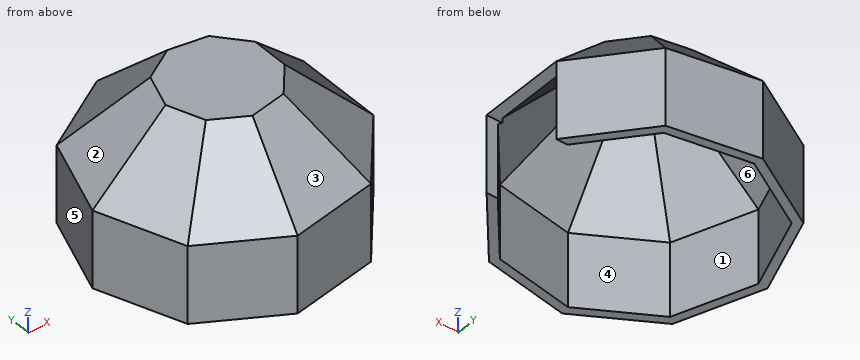
from build123d import *

# Parameters (mm, degrees)
F1_DEPTH = 85
F2_SIZE  = 40
F3_T     = -5
F4_W     = 50.557665
F4_H     = 45
F5_DEPTH = 70


with BuildPart() as f1:
    # F0 (on Top) → F1 (new body)
    with BuildSketch(Plane.XY):
        Polygon((-4.485587, -1.35111), (-4.485587, 49.206555), (-36.983427, 87.935973), (-86.773008, 96.715219), (-130.55723, 71.436387), (-147.84897, 23.927722), (-130.55723, -23.580943), (-86.773008, -48.859775), (-36.983427, -40.080529), align=None)
    extrude(amount=F1_DEPTH)

    # F2
    f2_edges = [f1.edges().sort_by_distance(p)[0] for p in [
        (-20.734507, -20.71582, 85),
        (-4.485587, 23.927722, 85),
        (-20.734507, 68.571264, 85),
        (-61.878218, 92.325596, 85),
        (-108.665119, 84.075803, 85),
        (-139.2031, 47.682054, 85),
        (-139.2031, 0.17339, 85),
        (-108.665119, -36.220359, 85),
        (-61.878218, -44.470152, 85),
    ]]
    chamfer(f2_edges, length=F2_SIZE)

    # F3
    f3_openings = [f1.faces().sort_by_distance(p)[0] for p in [
        (-73.938608, 23.927722, 0),
    ]]
    offset(amount=F3_T, openings=f3_openings)

    # F4 (on face) → F5 (cut)
    with BuildSketch(Plane.YZ.offset(-4.485587)):
        with Locations((23.927722, 22.5)):
            Rectangle(F4_W, F4_H)
    extrude(amount=-F5_DEPTH, mode=Mode.SUBTRACT)


solid = f1.part
Could you check a few things on this model? Use its own coordinates, in mm. Face numbers are marked on the shaded views. A direction names the side the tool comes from. Round coordinates to 2 decimals unless told otherwise and drop trailing zeros. Write each loop counter-clockwise with the first axis right and the second up, starting at its lowest first coordinate (ties: lowest second). Pieces come first, ordered by that corner, then holes. Notation, with made-up numbers: (4.5, 57.5) - (59.5, 57.5) arc R5 cw to (59.5, 61.5) - close; hole circle Ø11 at (88.5, -19.5). An arc over 180 degrees is marked (long way). Use a Markdown table: item, result.
Q1. I want a section at A-A (z = 64). List the corners of the cut face in (x, y) for me.
Output values:
| item | result |
|---|---|
| outline | (-127.63, 23.93) - (-115.07, -10.58) - (-83.26, -28.95) - (-47.09, -22.57) - (-23.49, 5.56) - (-23.49, 42.29) - (-47.09, 70.43) - (-83.26, 76.8) - (-115.07, 58.44) - close; hole (-120.1, 23.93) - (-109.3, -5.75) - (-81.96, -21.54) - (-50.86, -16.05) - (-30.56, 8.14) - (-30.56, 39.72) - (-50.86, 63.91) - (-81.96, 69.39) - (-109.3, 53.6) - close |
Q2. I want a section at C-C (z = 6.5). List the corners of the cut face in (x, y) for me, plus the area to 3 significant figures.
Output values:
| item | result |
|---|---|
| outline | (-147.85, 23.93) - (-130.56, -23.58) - (-86.77, -48.86) - (-36.98, -40.08) - (-4.49, -1.35) - (-11.01, -1.35) - (-39.64, -35.47) - (-85.85, -43.62) - (-126.48, -20.16) - (-142.53, 23.93) - (-126.48, 68.02) - (-85.85, 91.48) - (-39.64, 83.33) - (-11.01, 49.21) - (-4.49, 49.21) - (-36.98, 87.94) - (-86.77, 96.72) - (-130.56, 71.44) - close |
| area | 1,940 mm2 |
Q3. Thinking about a two-plate mould opening in Y: for the marked faces 1, 2, 3 and 4, which applies, released by +Y, released by -Y, zero draft, split by the parting line, or undercut?
Output values:
| item | result |
|---|---|
| face 1 | undercut |
| face 2 | released by +Y |
| face 3 | released by -Y |
| face 4 | undercut |
Q4. For pin 1 (6 mm diameter, centred on x = -48.5, z = 60, fed in from +Y); pin 2 (4 mm diameter, centred on x = -113, z = 17, fed in from -Y); pin 3 (8 mm diameter, centred on x = -104.5, y = 31, fed in from -Z), each with a flat end and sliding along its axis, tell me the tip position at first contact or that it passes through.
Output values:
| item | result |
|---|---|
| pin 1 | y = 77.83 |
| pin 2 | y = -34.87 |
| pin 3 | z = 72.24 |
Q5. Please list where these lines run through material, in increasing order: L1, parallel to Y at x = -91, z = 34; L2, parallel to X at y = -17, z = 5; L3, parallel to Y at x = -64.5, z = 61.
Output values:
| item | result |
|---|---|
| L1 | -46.42 to -40.65, 88.5 to 94.27 |
| L2 | -132.95 to -127.63, -24.14 to -17.62 |
| L3 | -28.69 to -21.51, 69.36 to 76.54 |
Q6. For the marked faces 5 and 6, which set-ups out of +Z, -Z, +X, -X, +Y, -Y let a thin tool reach every point of the face, with its end or its side?
Output values:
| item | result |
|---|---|
| face 5 | +Z, -Z, -X, +Y |
| face 6 | -Z |
Q7. I want a section at D-D (x = -67.5). List the corners of the cut face in (y, z) for me.
Output values:
| item | result |
|---|---|
| outline | (-45.46, 0) - (-40.38, 0) - (-40.38, 42.93) - (-2.74, 80) - (50.6, 80) - (88.24, 42.93) - (88.24, 0) - (93.32, 0) - (93.32, 45) - (52.7, 85) - (-4.84, 85) - (-45.46, 45) - close |
Q8. I want a section at B-B (y = -29). List the corners of the cut face in (x, z) for me.
Output values:
| item | result |
|---|---|
| outline | (-121.17, 0) - (-111.17, 0) - (-111.17, 42.93) - (-83.27, 56.88) - (-43.38, 49.95) - (-34.21, 42.93) - (-34.21, 0) - (-27.69, 0) - (-27.69, 45) - (-43.38, 57.02) - (-83.27, 63.95) - (-121.17, 45) - close |
